Read the model definition and answer for the solid it produces. Units are mm, in the model's axes. A direction names the side the tool comes from. Coordinates: 2 decimals unless noted, no trailing zeros. Order: outer loops, then holes, each group sorted by start corner. A loop starts at its lowest first (then second) coordinate and runs counter-clockwise, first axis right, second up.
```python
from build123d import *

# Parameters (mm, degrees)
EXTRUDE_2_DEPTH     = 5
SKETCH_4_R          = 1.65
CUT_EXTRUDE_1_DEPTH = 5
EXTRUDE_3_DEPTH     = 5
CUT_EXTRUDE_START   = -4.5
SKETCH_7_R          = 3
CUT_EXTRUDE_2_DEPTH = 3
CUT_EXTRUDE_3_DEPTH = 7.5
EXTRUDE_4_DEPTH     = 5
FILLET_1_R          = 5
FILLET_2_R          = 5
CUT_EXTRUDE_4_DEPTH = 5


with BuildPart() as part:
    # 草图3 → 凸台-拉伸2 (new body)
    with BuildSketch(Plane(origin=(0, 0, 0), x_dir=(1, 0, 0), z_dir=(0, 1, 0))):
        with BuildLine():
            Line((-3, -3.354101966), (-3, -7.416198487))
            Line((-3, -7.416198487), (-3, -43.854101966))
            Line((-3, -43.854101966), (3, -43.854101966))
            Line((3, -43.854101966), (3, -10.583005244))
            Line((3, -10.583005244), (3, -7.416198487))
            Line((3, -7.416198487), (3, -3.354101966))
            ThreePointArc((3, -3.354101966), (0, 4.5), (-3, -3.354101966))
        make_face()
    extrude(amount=EXTRUDE_2_DEPTH)

    # 草图4 → 切除-拉伸1 (cut)
    with BuildSketch(Plane(origin=(0, 5, 0), x_dir=(1, 0, 0), z_dir=(0, 1, 0))):
        with Locations(Location((0, 0, 0), (0, 0, 270))):
            Circle(SKETCH_4_R)
    extrude(amount=-CUT_EXTRUDE_1_DEPTH, mode=Mode.SUBTRACT)

    # 草图6 → 凸台-拉伸3 (add)
    with BuildSketch(Plane(origin=(0, 5, 0), x_dir=(1, 0, 0), z_dir=(0, 1, 0))):
        with BuildLine():
            Line((3, -33.74604712), (-3, -33.74604712))
            ThreePointArc((-3, -33.74604712), (-16.46902092, -57.986607816), (0.722500961, -79.745993902))
            Line((0.722500961, -79.745993902), (1.949520222, -77.620734201))
            ThreePointArc((1.949520222, -77.620734201), (-10.543317179, -55.371702353), (3, -33.74604712))
        make_face()
    extrude(amount=-EXTRUDE_3_DEPTH)

    # 草图7 → 切除-拉伸2 (cut)
    with BuildSketch(Plane(origin=(0, 5, 0), x_dir=(1, 0, 0), z_dir=(0, 1, 0)).offset(CUT_EXTRUDE_START)):
        with Locations(Location((0, 0, 0), (0, 0, 270))):
            Circle(SKETCH_7_R)
    extrude(amount=-CUT_EXTRUDE_2_DEPTH, mode=Mode.SUBTRACT)

    # 草图8 → 切除-拉伸3 (cut)
    with BuildSketch(Plane(origin=(0, 5, 0), x_dir=(1, 0, 0), z_dir=(0, 1, 0))):
        with BuildLine():
            Line((-3, -38.067187498), (-3, -43.854101966))
            Line((-3, -43.854101966), (3, -43.854101966))
            Line((3, -43.854101966), (3, -33.74604712))
            ThreePointArc((3, -33.74604712), (-0.160637142, -35.683569047), (-3, -38.067187498))
        make_face()
    extrude(amount=-CUT_EXTRUDE_3_DEPTH, mode=Mode.SUBTRACT)

    # 草图9 → 凸台-拉伸4 (add)
    with BuildSketch(Plane(origin=(0, 5, 0), x_dir=(1, 0, 0), z_dir=(0, 1, 0))):
        with BuildLine():
            Line((-3, -18.550074543), (-14.614967684, -46.324924269))
            ThreePointArc((-14.614967684, -46.324924269), (-9.917875534, -39.010182445), (-3, -33.74604712))
            Line((-3, -33.74604712), (-3, -18.550074543))
        make_face()
    extrude(amount=-EXTRUDE_4_DEPTH)

    # 圆角1
    fillet_1_edges = [part.edges().sort_by_distance(p)[0] for p in [
        (3, 2.5, 33.74604712),
    ]]
    fillet(fillet_1_edges, radius=FILLET_1_R)

    # 圆角2
    # the kernel refuses this fillet: 5 mm, written as the material it takes off along each edge
    with BuildSketch(Plane(origin=(1.949520222, 14.371610933, 77.620734201), x_dir=(-0.8261015944022844, 0, -0.5635212114250925), z_dir=(0, -1, 0))) as fillet_2_piece_1:
        with BuildLine():
            CenterArc((4.123508811, -4.985927863), FILLET_2_R, 94.299664485, 55.185648669)
            Line((-0.183986354, -2.447131808), (-0.270136257, -2.396355887))
            ThreePointArc((-0.270136257, -2.396355887), (-0.191711734, -1.216068615), (-0.099718557, 0.007497289))
            Line((-0.099718557, 0.007497289), (0.007497289, 0.099718557))
            ThreePointArc((0.007497289, 0.099718557), (1.874322187, 0.029639314), (3.741147084, 0.099718557))
            Line((3.741147084, 0.099718557), (3.748644373, 0))
        make_face()
    extrude(amount=23.743221866, mode=Mode.SUBTRACT)

    # 草图10 → 切除-拉伸4 (cut)
    with BuildSketch(Plane(origin=(0, 5, 0), x_dir=(1, 0, 0), z_dir=(0, 1, 0))):
        with BuildLine():
            Line((-14.614967684, -46.324924269), (-8.614967684, -46.324924269))
            ThreePointArc((-8.614967684, -46.324924269), (-9.770106213, -62.167654699), (-1.147240872, -75.508293582))
            ThreePointArc((-1.147240872, -75.508293582), (0.307928877, -77.397579493), (0.722500961, -79.745993902))
            ThreePointArc((0.722500961, -79.745993902), (-14.272081884, -66.397409294), (-14.614967684, -46.324924269))
        make_face()
    extrude(amount=-CUT_EXTRUDE_4_DEPTH, mode=Mode.SUBTRACT)


solid = part.part
```
1) A cutting plane is placed at A-A, the plane y = 2.95. Determine the outline of the cut face in (x, z).
A:
outline: (-14.61, 46.32) - (-3, 18.55) - (-3, 3.35) arc R4.5 ccw (long way) to (3, 3.35) - (3, 30.88) arc R5 ccw to (0.74, 35.06) arc R25 cw to (-8.61, 46.32) - close; hole circle Ø3.3 at (0, 0)
2) Determine the mould class of faces 1 (the flat face through (-1.3, 0.5, 1.3)), 2 (the cylindrical face through (2.416, 2.465, 33.228)), 3 (the flat face through (-3, 2, 11)), 4 (the flat face through (3, 2, 17)) for opening direction Z: pulls with the +Z half, pulls with the -Z half, needs draft (parallel to the pull), parting line crosses it, or undercut.
A:
face 1: undercut
face 2: pulls with the +Z half
face 3: undercut
face 4: needs draft
3) A cutting plane is placed at D-D, the plane z = 28.5. Determine the outline of the cut face in (x, y), and give its area (3 significant figures).
A:
outline: (-7.16, 0) - (3, 0) - (3, 5) - (-7.16, 5) - close
area: 50.8 mm2
4) A cutting plane is placed at B-B, the plane z = 0. Determine the outline of the cut face in (x, y), and give its area (4 significant figures).
A:
outline: (-4.5, 0) - (-3, 0) - (-3, 0.5) - (-1.65, 0.5) - (-1.65, 5) - (-4.5, 5) - close; (1.65, 0.5) - (3, 0.5) - (3, 0) - (4.5, 0) - (4.5, 5) - (1.65, 5) - close
area: 27.15 mm2
5) Straight lines are drawn through the part: line 1 (X direction, y = 0.3, z = 0); line 2 (X direction, y = 1.7, z = 0); line 3 (X direction, y = 0.4, z = 12). For each, find the intervals that lie inside material, in ascending order.
A:
line 1: x = -4.5 to -3, 3 to 4.5
line 2: x = -4.5 to -1.65, 1.65 to 4.5
line 3: x = -3 to 3
6) Flat-ended cylindrical pins translate along their axes: pin 1 Ø3 at (x, z) = (0, 0) entering from -Y; pin 2 Ø3 at (x, y) = (-2, 1.5) entering from -Z; pin 3 Ø1.5 at (y, z) = (3, 12) entering from -X; pin 4 Ø1 at (x, y) = (-6.5, 4) entering from +Z. Find the tip coordinate at first contact, or state that the pin passes through.
A:
pin 1: passes through
pin 2: stops at z = -4.47
pin 3: stops at x = -3
pin 4: stops at z = 43.13
7) A cutting plane is placed at C-C, the plane x = 0. Determine the outline of the cut face in (y, z).
A:
outline: (0, -4.5) - (5, -4.5) - (5, -1.65) - (0.5, -1.65) - (0.5, -3) - (0, -3) - close; (0, 3) - (0.5, 3) - (0.5, 1.65) - (5, 1.65) - (5, 35.57) - (0, 35.57) - close
8) Which of the six approach directions +Z, -Z, +X, -X, +Y, -Y give full straight-line access (tool end or side, diameter ignored) to faces 5 (the cylindrical face through (0.9, 0.25, 2.86)), 6 (the flat face through (-12, 3, 46.325))?
A:
face 5: -Y
face 6: +Z, +X, -X, +Y, -Y
